The model under review builds one solid part; all positions refer to its coordinate system, in mm. A direction names the side the tool comes from. Round coordinates to 2 decimals unless told otherwise and drop trailing zeros. Loops run counter-clockwise (first coordinate to the right, second up) from the corner with the lowest first, then second, coordinate; pieces in that order, holes last. Notation, with made-up numbers: (73.5, -29.75) -> (127.5, -29.75) arc R28 cw to (127.5, 4.25) -> close; hole circle Ø3 at (75, 51). An arc over 180 degrees is marked (long way). Return JSON: item names as keys, results as strings. Group by question number.
```python
from build123d import *

# Parameters (mm, degrees)
F0_R     = 12
F0_R_2   = 10
F1_DEPTH = 30
F0_R_3   = 21
F2_DEPTH = 20.5
F3_DEPTH = 22
F0_R_4   = 6
F4_DEPTH = 20.5
F5_DEPTH = 7
F6_DEPTH = 5


with BuildPart() as f1:
    # F0 (on Right) → F1 (new body)
    with BuildSketch(Plane.YZ):
        Circle(F0_R)
        Circle(F0_R_2, mode=Mode.SUBTRACT)
    extrude(amount=F1_DEPTH)

    # F0 (on Right) → F2 (join)
    with BuildSketch(Plane.YZ):
        with BuildLine():
            ThreePointArc((-8.0963332733, 23.6526824594), (-17.6776695297, 17.6776695297), (-23.6526824594, 8.0963332733))
            Line((-23.6526824594, 8.0963332733), (-22.0610314501, 6.504682264))
            ThreePointArc((-22.0610314501, 6.504682264), (-23, -4.4e-09), (-22.0610314476, -6.5046822725))
            Line((-22.0610314476, -6.5046822725), (-23.6526824563, -8.0963332824))
            ThreePointArc((-23.6526824563, -8.0963332824), (-17.6776695229, -17.6776695365), (-8.0963332642, -23.6526824626))
            Line((-8.0963332642, -23.6526824626), (-6.5046822555, -22.0610314526))
            ThreePointArc((-6.5046822555, -22.0610314526), (7.4e-09, -23), (6.5046822697, -22.0610314485))
            Line((6.5046822697, -22.0610314485), (8.0963332794, -23.6526824574))
            ThreePointArc((8.0963332794, -23.6526824574), (17.6776695342, -17.6776695251), (23.6526824615, -8.0963332673))
            Line((23.6526824615, -8.0963332673), (22.0610314518, -6.5046822584))
            ThreePointArc((22.0610314518, -6.5046822584), (23, 4.4e-09), (22.0610314493, 6.5046822669))
            Line((22.0610314493, 6.5046822669), (23.6526824584, 8.0963332764))
            ThreePointArc((23.6526824584, 8.0963332764), (17.6776695274, 17.6776695319), (8.0963332703, 23.6526824605))
            Line((8.0963332703, 23.6526824605), (6.5046822612, 22.061031451))
            ThreePointArc((6.5046822612, 22.061031451), (-1.5e-09, 23), (-6.504682264, 22.0610314501))
            Line((-6.504682264, 22.0610314501), (-8.0963332733, 23.6526824594))
        make_face()
        Circle(F0_R_3, mode=Mode.SUBTRACT)
        Circle(F0_R_3)
        Circle(F0_R, mode=Mode.SUBTRACT)
    extrude(amount=F2_DEPTH)

    # F0 (on Right) → F3 (join)
    with BuildSketch(Plane.YZ):
        with BuildLine():
            Line((-22.0610314501, 6.504682264), (-23.6526824594, 8.0963332733))
            ThreePointArc((-23.6526824594, 8.0963332733), (-25, -4.8e-09), (-23.6526824563, -8.0963332824))
            Line((-23.6526824563, -8.0963332824), (-22.0610314476, -6.5046822725))
            ThreePointArc((-22.0610314476, -6.5046822725), (-23, -4.4e-09), (-22.0610314501, 6.504682264))
        make_face()
        with BuildLine():
            ThreePointArc((8.0963332703, 23.6526824605), (-1.6e-09, 25), (-8.0963332733, 23.6526824594))
            Line((-8.0963332733, 23.6526824594), (-6.504682264, 22.0610314501))
            ThreePointArc((-6.504682264, 22.0610314501), (-1.5e-09, 23), (6.5046822612, 22.061031451))
            Line((6.5046822612, 22.061031451), (8.0963332703, 23.6526824605))
        make_face()
        with BuildLine():
            ThreePointArc((25, 0), (24.6608704374, 4.1038359214), (23.6526824584, 8.0963332764))
            Line((23.6526824584, 8.0963332764), (22.0610314493, 6.5046822669))
            ThreePointArc((22.0610314493, 6.5046822669), (23, 4.4e-09), (22.0610314518, -6.5046822584))
            Line((22.0610314518, -6.5046822584), (23.6526824615, -8.0963332673))
            ThreePointArc((23.6526824615, -8.0963332673), (24.6608704382, -4.1038359167), (25, 0))
        make_face()
        with BuildLine():
            Line((-6.5046822555, -22.0610314526), (-8.0963332642, -23.6526824626))
            ThreePointArc((-8.0963332642, -23.6526824626), (8e-09, -25), (8.0963332794, -23.6526824574))
            Line((8.0963332794, -23.6526824574), (6.5046822697, -22.0610314485))
            ThreePointArc((6.5046822697, -22.0610314485), (7.4e-09, -23), (-6.5046822555, -22.0610314526))
        make_face()
    extrude(amount=F3_DEPTH)

    # F0 (on Right) → F4 (join, through all)
    with BuildSketch(Plane.YZ):
        with BuildLine():
            Line((-35.3553390593, 19.7989898732), (-23.6526824594, 8.0963332733))
            ThreePointArc((-23.6526824594, 8.0963332733), (-17.6776695297, 17.6776695297), (-8.0963332733, 23.6526824594))
            Line((-8.0963332733, 23.6526824594), (-19.7989898732, 35.3553390593))
            ThreePointArc((-19.7989898732, 35.3553390593), (-27.5771644248, 38.5771644663), (-35.3553390007, 35.355339118))
            ThreePointArc((-35.3553390007, 35.355339118), (-38.5771644663, 27.5771645077), (-35.3553390593, 19.7989898732))
        make_face()
        with Locations((-27.5771644663, 27.5771644663)):
            Circle(F0_R_4, mode=Mode.SUBTRACT)
        with BuildLine():
            ThreePointArc((-8.0963332642, -23.6526824626), (-17.6776695229, -17.6776695365), (-23.6526824563, -8.0963332824))
            Line((-23.6526824563, -8.0963332824), (-35.3553390517, -19.7989898868))
            ThreePointArc((-35.3553390517, -19.7989898868), (-38.5771644557, -27.5771644811), (-35.3553390457, -35.3553390729))
            ThreePointArc((-35.3553390457, -35.3553390729), (-27.5771644514, -38.5771644769), (-19.7989898596, -35.3553390669))
            Line((-19.7989898596, -35.3553390669), (-8.0963332642, -23.6526824626))
        make_face()
        with Locations((-27.5771644557, -27.5771644769)):
            Circle(F0_R_4, mode=Mode.SUBTRACT)
        with BuildLine():
            ThreePointArc((23.6526824615, -8.0963332673), (17.6776695342, -17.6776695251), (8.0963332794, -23.6526824574))
            Line((8.0963332794, -23.6526824574), (19.7989898823, -35.3553390542))
            ThreePointArc((19.7989898823, -35.3553390542), (27.5771645176, -38.5771644592), (35.355339127, -35.3553389916))
            ThreePointArc((35.355339127, -35.3553389916), (38.5771644733, -27.5771644149), (35.3553390644, -19.7989898642))
            Line((35.3553390644, -19.7989898642), (23.6526824615, -8.0963332673))
        make_face()
        with Locations((27.5771644733, -27.5771644592)):
            Circle(F0_R_4, mode=Mode.SUBTRACT)
        with BuildLine():
            Line((19.7989898687, 35.3553390619), (8.0963332703, 23.6526824605))
            ThreePointArc((8.0963332703, 23.6526824605), (17.6776695274, 17.6776695319), (23.6526824584, 8.0963332764))
            Line((23.6526824584, 8.0963332764), (35.3553390568, 19.7989898778))
            ThreePointArc((35.3553390568, 19.7989898778), (38.5771644627, 27.5771644712), (35.3553390548, 35.3553390639))
            ThreePointArc((35.3553390548, 35.3553390639), (27.5771644613, 38.5771644698), (19.7989898687, 35.3553390619))
        make_face()
        with Locations((27.5771644627, 27.5771644698)):
            Circle(F0_R_4, mode=Mode.SUBTRACT)
    extrude(amount=F4_DEPTH)

    # F0 (on Right) → F5 (join)
    with BuildSketch(Plane.YZ):
        with BuildLine():
            ThreePointArc((-23.6526824563, -8.0963332824), (-25, -4.8e-09), (-23.6526824594, 8.0963332733))
            Line((-23.6526824594, 8.0963332733), (-35.3553390593, 19.7989898732))
            ThreePointArc((-35.3553390593, 19.7989898732), (-38.5771644663, 27.5771645077), (-35.3553390007, 35.355339118))
            ThreePointArc((-35.3553390007, 35.355339118), (-50, 3.19e-08), (-35.3553390457, -35.3553390729))
            ThreePointArc((-35.3553390457, -35.3553390729), (-38.5771644557, -27.5771644811), (-35.3553390517, -19.7989898868))
            Line((-35.3553390517, -19.7989898868), (-23.6526824563, -8.0963332824))
        make_face()
        with BuildLine():
            Line((-19.7989898732, 35.3553390593), (-8.0963332733, 23.6526824594))
            ThreePointArc((-8.0963332733, 23.6526824594), (-1.6e-09, 25), (8.0963332703, 23.6526824605))
            Line((8.0963332703, 23.6526824605), (19.7989898687, 35.3553390619))
            ThreePointArc((19.7989898687, 35.3553390619), (27.5771644613, 38.5771644698), (35.3553390548, 35.3553390639))
            ThreePointArc((35.3553390548, 35.3553390639), (3.83e-08, 50), (-35.3553390007, 35.355339118))
            ThreePointArc((-35.3553390007, 35.355339118), (-27.5771644248, 38.5771644663), (-19.7989898732, 35.3553390593))
        make_face()
        with BuildLine():
            ThreePointArc((8.0963332794, -23.6526824574), (8e-09, -25), (-8.0963332642, -23.6526824626))
            Line((-8.0963332642, -23.6526824626), (-19.7989898596, -35.3553390669))
            ThreePointArc((-19.7989898596, -35.3553390669), (-27.5771644514, -38.5771644769), (-35.3553390457, -35.3553390729))
            ThreePointArc((-35.3553390457, -35.3553390729), (5.75e-08, -50), (35.355339127, -35.3553389916))
            ThreePointArc((35.355339127, -35.3553389916), (27.5771645176, -38.5771644592), (19.7989898823, -35.3553390542))
            Line((19.7989898823, -35.3553390542), (8.0963332794, -23.6526824574))
        make_face()
        with BuildLine():
            ThreePointArc((50, 0), (46.1939766243, 19.1341716212), (35.3553390548, 35.3553390639))
            ThreePointArc((35.3553390548, 35.3553390639), (38.5771644627, 27.5771644712), (35.3553390568, 19.7989898778))
            Line((35.3553390568, 19.7989898778), (23.6526824584, 8.0963332764))
            ThreePointArc((23.6526824584, 8.0963332764), (24.6608704374, 4.1038359214), (25, 0))
            ThreePointArc((25, 0), (24.6608704382, -4.1038359167), (23.6526824615, -8.0963332673))
            Line((23.6526824615, -8.0963332673), (35.3553390644, -19.7989898642))
            ThreePointArc((35.3553390644, -19.7989898642), (38.5771644733, -27.5771644149), (35.355339127, -35.3553389916))
            ThreePointArc((35.355339127, -35.3553389916), (46.1939766439, -19.134171574), (50, 0))
        make_face()
    extrude(amount=F5_DEPTH)

    # F0 (on Right) → F6 (join)
    with BuildSketch(Plane.YZ):
        with BuildLine():
            ThreePointArc((-8.0963332733, 23.6526824594), (-17.6776695297, 17.6776695297), (-23.6526824594, 8.0963332733))
            Line((-23.6526824594, 8.0963332733), (-22.0610314501, 6.504682264))
            ThreePointArc((-22.0610314501, 6.504682264), (-23, -4.4e-09), (-22.0610314476, -6.5046822725))
            Line((-22.0610314476, -6.5046822725), (-23.6526824563, -8.0963332824))
            ThreePointArc((-23.6526824563, -8.0963332824), (-17.6776695229, -17.6776695365), (-8.0963332642, -23.6526824626))
            Line((-8.0963332642, -23.6526824626), (-6.5046822555, -22.0610314526))
            ThreePointArc((-6.5046822555, -22.0610314526), (7.4e-09, -23), (6.5046822697, -22.0610314485))
            Line((6.5046822697, -22.0610314485), (8.0963332794, -23.6526824574))
            ThreePointArc((8.0963332794, -23.6526824574), (17.6776695342, -17.6776695251), (23.6526824615, -8.0963332673))
            Line((23.6526824615, -8.0963332673), (22.0610314518, -6.5046822584))
            ThreePointArc((22.0610314518, -6.5046822584), (23, 4.4e-09), (22.0610314493, 6.5046822669))
            Line((22.0610314493, 6.5046822669), (23.6526824584, 8.0963332764))
            ThreePointArc((23.6526824584, 8.0963332764), (17.6776695274, 17.6776695319), (8.0963332703, 23.6526824605))
            Line((8.0963332703, 23.6526824605), (6.5046822612, 22.061031451))
            ThreePointArc((6.5046822612, 22.061031451), (-1.5e-09, 23), (-6.504682264, 22.0610314501))
            Line((-6.504682264, 22.0610314501), (-8.0963332733, 23.6526824594))
        make_face()
        Circle(F0_R_3, mode=Mode.SUBTRACT)
        with BuildLine():
            Line((-22.0610314501, 6.504682264), (-23.6526824594, 8.0963332733))
            ThreePointArc((-23.6526824594, 8.0963332733), (-25, -4.8e-09), (-23.6526824563, -8.0963332824))
            Line((-23.6526824563, -8.0963332824), (-22.0610314476, -6.5046822725))
            ThreePointArc((-22.0610314476, -6.5046822725), (-23, -4.4e-09), (-22.0610314501, 6.504682264))
        make_face()
        with BuildLine():
            ThreePointArc((8.0963332703, 23.6526824605), (-1.6e-09, 25), (-8.0963332733, 23.6526824594))
            Line((-8.0963332733, 23.6526824594), (-6.504682264, 22.0610314501))
            ThreePointArc((-6.504682264, 22.0610314501), (-1.5e-09, 23), (6.5046822612, 22.061031451))
            Line((6.5046822612, 22.061031451), (8.0963332703, 23.6526824605))
        make_face()
        with BuildLine():
            ThreePointArc((25, 0), (24.6608704374, 4.1038359214), (23.6526824584, 8.0963332764))
            Line((23.6526824584, 8.0963332764), (22.0610314493, 6.5046822669))
            ThreePointArc((22.0610314493, 6.5046822669), (23, 4.4e-09), (22.0610314518, -6.5046822584))
            Line((22.0610314518, -6.5046822584), (23.6526824615, -8.0963332673))
            ThreePointArc((23.6526824615, -8.0963332673), (24.6608704382, -4.1038359167), (25, 0))
        make_face()
        with BuildLine():
            Line((-6.5046822555, -22.0610314526), (-8.0963332642, -23.6526824626))
            ThreePointArc((-8.0963332642, -23.6526824626), (8e-09, -25), (8.0963332794, -23.6526824574))
            Line((8.0963332794, -23.6526824574), (6.5046822697, -22.0610314485))
            ThreePointArc((6.5046822697, -22.0610314485), (7.4e-09, -23), (-6.5046822555, -22.0610314526))
        make_face()
    extrude(amount=-F6_DEPTH)


solid = f1.part
```
1. Draft analysis for pull direction Y (two halves, no side actions). For faces 1 (the face through (7, -37, 0)), 2 (the face through (14, 0, 25)), 3 (the face through (13.656, -29.586, 14.03)), state which applies: pulls with the +Y half, pulls with the -Y half, needs draft (parallel to the pull), parting line crosses it, or undercut.
2. Wall thickness on line 1 (Z direction, x = 18, y = 27); line 2 (Y direction, x = 6.5, z = 32); line 3 (Z direction, x = 8, y = -23): over which ranges is each line inside the solid? List them lowest first.
3. We need section C-C, the plane x = 17. Write out the cut boundary in (y, z).
4. We need section B-B, the plane z = -2. Write out the cut boundary in (x, y), then the cut area to 3 significant figures.
5. We need section D-D, the plane y = -31. Write out the cut boundary in (x, z), then the cut area to 3 significant figures.
6. Tool access review of faces 4 (the face through (22, 0, -24)), 5 (the face through (14, 0, -25)), 6 (the face through (22, -24, 0)), 7 (the face through (22, 24, 0)), 8 (the face through (20.5, -9, 9)): name each direction out of +Z, -Z, +X, -X, +Y, -Y from which nothing blocks a thin tool from reaching the whole face with its end or side.
7. For P1, Ø8, axis at x = 10, y = 37, coming from the -Z side; P2, Ø15.5, axis at y = 27.58, z = -27.58, coming from the +X side; P3, Ø15.5, axis at y = -27.58, z = 27.58, coming from the -X side; P4, Ø25, axis at y = 0, z = 0, coming from the +X side, all flat-tipped, find the tip position at first contact; note any pin that passes through.
8. We need section A-A, the plane y = 0. Write out the cut boundary in (x, z), then the cut area to 3 significant figures.
Check sheet entries:
{
 "1": {"face 1": "needs draft", "face 2": "undercut", "face 3": "pulls with the -Y half"},
 "2": {"line 1": "z = -38.56 to -33.55, -21.6 to -11.44, 11.44 to 21.6, 33.55 to 38.56", "line 2": "y = -38.42 to -31.63, -23.52 to 23.52, 31.63 to 38.42", "line 3": "z = -37.58 to -31.46, -23.7 to 23.7, 31.46 to 37.58"},
 "3": {"outline": "(-35.36, -19.8) arc R11 ccw to (-19.8, -35.36) -> (-8.1, -23.65) arc R25 ccw to (8.1, -23.65) -> (19.8, -35.36) arc R11 ccw to (35.36, -19.8) -> (23.65, -8.1) arc R25 ccw to (23.65, 8.1) -> (35.36, 19.8) arc R11 ccw to (19.8, 35.36) -> (8.1, 23.65) arc R25 ccw to (-8.1, 23.65) -> (-19.8, 35.36) arc R11 ccw to (-35.36, 19.8) -> (-23.65, 8.1) arc R25 ccw to (-23.65, -8.1) -> close; hole circle Ø12 at (-27.58, -27.58); hole circle Ø12 at (-27.58, 27.58); hole circle Ø20 at (0, 0); hole circle Ø12 at (27.58, -27.58); hole circle Ø12 at (27.58, 27.58)"},
 "4": {"outline": "(-5, -24.92) -> (0, -24.92) -> (0, -49.96) -> (7, -49.96) -> (7, -24.92) -> (22, -24.92) -> (22, -22.91) -> (20.5, -22.91) -> (20.5, -11.83) -> (30, -11.83) -> (30, -9.8) -> (0, -9.8) -> (0, -20.9) -> (-5, -20.9) -> close; (-5, 20.9) -> (0, 20.9) -> (0, 9.8) -> (30, 9.8) -> (30, 11.83) -> (20.5, 11.83) -> (20.5, 22.91) -> (22, 22.91) -> (22, 24.92) -> (7, 24.92) -> (7, 49.96) -> (0, 49.96) -> (0, 24.92) -> (-5, 24.92) -> close", "area": "1,060 mm²"},
 "5": {"outline": "(0, -39.23) -> (7, -39.23) -> (7, -38.03) -> (20.5, -38.03) -> (20.5, -32.51) -> (0, -32.51) -> close; (0, -22.65) -> (20.5, -22.65) -> (20.5, -15.44) -> (7, -15.44) -> (7, 15.44) -> (20.5, 15.44) -> (20.5, 22.65) -> (0, 22.65) -> close; (0, 32.51) -> (20.5, 32.51) -> (20.5, 38.03) -> (7, 38.03) -> (7, 39.23) -> (0, 39.23) -> close", "area": "755 mm²"},
 "6": {"face 4": "-Z, +X, +Y, -Y", "face 5": "-Z, +X", "face 6": "+Z, -Z, +X, -Y", "face 7": "+Z, -Z, +X, +Y", "face 8": "+X"},
 "7": {"P1": "stops at z = -37.15", "P2": "stops at x = 20.5", "P3": "stops at x = 0", "P4": "stops at x = 30"},
 "8": {"outline": "(-5, -25) -> (0, -25) -> (0, -50) -> (7, -50) -> (7, -25) -> (22, -25) -> (22, -23) -> (20.5, -23) -> (20.5, -12) -> (30, -12) -> (30, -10) -> (0, -10) -> (0, -21) -> (-5, -21) -> close; (-5, 21) -> (0, 21) -> (0, 10) -> (30, 10) -> (30, 12) -> (20.5, 12) -> (20.5, 23) -> (22, 23) -> (22, 25) -> (7, 25) -> (7, 50) -> (0, 50) -> (0, 25) -> (-5, 25) -> close", "area": "1,050 mm²"}
}
